For this review, take the finished solid that the model builds, in its own axes (mm). A direction names the side the tool comes from. Coordinates: 2 decimals unless noted, no trailing zeros. Write each loop counter-clockwise with the first axis right and the second up, starting at its lowest first coordinate (ties: lowest second). Pieces come first, ordered by that corner, then holes.
1) Mouldability with a two-part tool opening along Z and no side actions: class faces 3 (the face through (14, -49, -500)), 4 (the face through (-899, -1100, -399)), 5 (the face through (-947.69, -593, -384.98)) as pulls with the +Z half, pulls with the -Z half, needs draft (parallel to the pull), parting line crosses it, or undercut.
2) To check wall thickness, follow line 1 along Y through (x, z) = (-833, -66); line 2 along Z through (x, y) = (856.5, -517); line 3 along X through (y, z) = (-939.5, 376). State the ranges of each line that lie inside material, in increasing order.
3) We need section B-B on x = -900. Write out the cut boundary in (y, z), then the cut area to 3 significant figures.
4) We need section A-A on z = 400. Write out the cut boundary in (x, y), then the cut area to 3 significant figures.
5) We need section D-D on z = 174. Write out the cut boundary in (x, y), then the cut area to 3 significant figures.
6) We need section C-C on y = -345. Write out the cut boundary in (x, z).
7) For faces 1 (the face through (1000, -49, -7)), 2 (the face through (947.69, -593, -384.98)), list the 3-axis set-ups (+Z, -Z, +X, -X, +Y, -Y) from which the entire face can be reached by the end or side of a thin tool; tool diameter is ignored.
8) Insertion check: P1, Ø1, axis at x = 88, z = -13, coming from the -Y side; P2, Ø1, axis at y = -313, z = 374, coming from the +X side; P3, Ø5, axis at x = -156.5, z = -399.5, coming from the +Y side. Each pin has a flat end and moves straight along its axis. Give the tip position at first contact, or say it passes through.
from build123d import *

# Parameters (mm, degrees)
SKETCH1_W               = 1000
SKETCH1_H               = 500
BOSS_EXTRUDE1_DEPTH     = 100
SKETCH2_R               = 50
BOSS_EXTRUDE2_DEPTH     = 1000
MIRROR2_COPY_1_SKETCH_W = 1000
MIRROR2_COPY_1_SKETCH_H = 500
MIRROR2_COPY_1_DEPTH    = 100
MIRROR2_COPY_2_SKETCH_R = 50
MIRROR2_COPY_2_DEPTH    = 1000


with BuildPart() as part:
    # Sketch1 → Boss-Extrude1 (new body)
    with BuildSketch(Plane(origin=(0, 0, 0), x_dir=(1, 0, 0), z_dir=(0, 1, 0))):
        with Locations((500, 250)):
            Rectangle(SKETCH1_W, SKETCH1_H)
    boss_extrude1 = extrude(amount=-BOSS_EXTRUDE1_DEPTH)

    # Sketch2 → Boss-Extrude2 (add)
    with BuildSketch(Plane.XZ.offset(100)):
        with Locations((900, -400)):
            Circle(SKETCH2_R)
    boss_extrude2 = extrude(amount=BOSS_EXTRUDE2_DEPTH)

    # Mirror1: Boss-Extrude1, Boss-Extrude2 across plane
    add(boss_extrude1.mirror(Plane(origin=(0, 0, 0), x_dir=(0, 0, 1), z_dir=(1, 0, 0))))
    add(boss_extrude2.mirror(Plane(origin=(0, 0, 0), x_dir=(0, 0, 1), z_dir=(1, 0, 0))))

    # Mirror2: Boss-Extrude2, Boss-Extrude1 across plane
    add(boss_extrude2.mirror(Plane.XY))
    add(boss_extrude1.mirror(Plane.XY))

    # Mirror2 copy 1 sketch → Mirror2 copy 1 (add)
    with BuildSketch(Plane(origin=(0, 0, 0), x_dir=(-1, 0, 0), z_dir=(0, 1, 0))):
        with Locations((500, 250)):
            Rectangle(MIRROR2_COPY_1_SKETCH_W, MIRROR2_COPY_1_SKETCH_H)
    extrude(amount=-MIRROR2_COPY_1_DEPTH)

    # Mirror2 copy 2 sketch → Mirror2 copy 2 (add)
    with BuildSketch(Plane(origin=(0, -100, 0), x_dir=(-1, 0, 0), z_dir=(0, -1, 0))):
        with Locations((900, -400)):
            Circle(MIRROR2_COPY_2_SKETCH_R)
    extrude(amount=MIRROR2_COPY_2_DEPTH)


solid = part.part
Result:
1. face 3: pulls with the -Z half
1. face 4: needs draft
1. face 5: undercut
2. line 1: y = -100 to 0
2. line 2: z = -424.65 to -375.35, 375.35 to 424.65
2. line 3: x = -943.86 to -856.14, 856.14 to 943.86
3. outline: (-1100, -450) - (-100, -450) - (-100, -500) - (0, -500) - (0, 500) - (-100, 500) - (-100, 450) - (-1100, 450) - (-1100, 350) - (-100, 350) - (-100, -350) - (-1100, -350) - close
3. area: 300,000 mm2
4. outline: (-1000, -100) - (-950, -100) - (-950, -1100) - (-850, -1100) - (-850, -100) - (850, -100) - (850, -1100) - (950, -1100) - (950, -100) - (1000, -100) - (1000, 0) - (-1000, 0) - close
4. area: 400,000 mm2
5. outline: (-1000, -100) - (1000, -100) - (1000, 0) - (-1000, 0) - close
5. area: 200,000 mm2
6. outline: circle Ø100 at (-900, -400); circle Ø100 at (-900, 400); circle Ø100 at (900, -400); circle Ø100 at (900, 400)
7. face 1: +Z, -Z, +X, +Y, -Y
7. face 2: -Y
8. P1: stops at y = -100
8. P2: stops at x = 943.01
8. P3: stops at y = 0
